The listing builds one solid part. Answer for the finished solid, in the listing's coordinates (mm). A direction names the side the tool comes from. Give positions to 0.01 mm unless a question says otherwise; leave off trailing zeros. Write each loop counter-clockwise with the first axis right and the second up, starting at its lowest first coordinate (ties: lowest second). Pieces come first, ordered by that corner, then holes. Notation, with made-up numbers: (43, -21.75) -> (81, -21.75) arc R26 cw to (81, 14.25) -> close; hole circle Ø7 at (4, -32.75). An arc over 180 degrees is marked (long way). Put each result on its own line as item: value. Start each with the question number.
1) For faces 3 (the flat face through (378.107, 102.08, 85.404)), 4 (the cylindrical face through (466.41, 102.92, 207.94)), 5 (the cylindrical face through (453.3, 102.08, 231.05)), determine the directions among +Z, -Z, +X, -X, +Y, -Y from which every point of the face is accessible in a straight line to the end or side of a thin tool.
2) A cutting plane is placed at D-D (y = 23). Write down the section's boundary in (x, z).
3) A cutting plane is placed at C-C (x = 663.5). Write down the section's boundary in (y, z), then the cut area to 3 significant figures.
4) For a pull along Y with two mould halves and no side action, classify faces 1 (the flat face through (-300, 75, 101)), 2 (the flat face through (423, 132.5, 120)) as released by +Y, released by -Y, zero draft, split by the parting line, or undercut.
5) A cutting plane is placed at A-A (y = 114.5). Give the number of separate pieces and of enclosed holes in the cut face, then the cut area to 3 significant figures.
6) A cutting plane is placed at B-B (z = 232.5). Write down the section's boundary in (x, y).
7) Flat-ended cylindrical pins translate along their axes: pin 1 Ø22 at (x, y) = (556.5, 144.5) entering from -Z; pin 2 Ø4 at (y, z) = (72, 204) entering from -X; pin 3 Ø18 at (x, y) = (586, 106) entering from -Z. Find the tip coordinate at first contact, or state that the pin passes through.
8) Find the intervals of material crossed by line 1 along Y through (x, z) = (500, 195.5); line 2 along X through (y, z) = (118.5, 232.5); line 3 along Z through (x, y) = (652, 66), in increasing order. Write a range as from..to.
from build123d import *

# Parameters (mm, degrees)
BOSS_EXTRUDE1_DEPTH = 152.5
CUT_EXTRUDE1_DEPTH  = 153.5
CUT_EXTRUDE2_REACH  = 154.5
SKETCH7_R           = 35


with BuildPart() as part:
    # Sketch1 → Boss-Extrude1 (new body)
    with BuildSketch(Plane(origin=(0, 0, 0), x_dir=(1, 0, 0), z_dir=(0, 1, 0))):
        with BuildLine():
            Line((-300, -132.5), (-132.5, -132.5))
            ThreePointArc((-132.5, -132.5), (-38.808351493, -93.691648507), (0, 0))
            Line((0, 0), (0, 209.763098819))
            ThreePointArc((0, 209.763098819), (-38.808351493, 303.454747326), (-132.5, 342.263098819))
            Line((-132.5, 342.263098819), (-300, 342.263098819))
            Line((-300, 342.263098819), (-300, 279.881549409))
            Line((-300, 279.881549409), (-125, 104.881549409))
            Line((-125, 104.881549409), (-300, -70.118450591))
            Line((-300, -70.118450591), (-300, -132.5))
        make_face()
    extrude(amount=BOSS_EXTRUDE1_DEPTH)

    # Sketch2 → Cut-Extrude1 (cut, through all)
    with BuildSketch(Plane(origin=(0, 152.5, 0), x_dir=(1, 0, 0), z_dir=(0, 1, 0))):
        with BuildLine():
            Line((-223.447835998, -46.182307711), (-139.361825834, 46.305891731))
            ThreePointArc((-139.361825834, 46.305891731), (-95.697655057, 48.504400086), (-93.258215037, 4.853026901))
            Line((-93.258215037, 4.853026901), (-176.318308109, -88.557599262))
            ThreePointArc((-176.318308109, -88.557599262), (-221.187968417, -91.065122785), (-223.447835998, -46.182307711))
        make_face()
        with BuildLine():
            Line((-93.258215037, 204.910071918), (-176.318308109, 298.320698081))
            ThreePointArc((-176.318308109, 298.320698081), (-221.187968417, 300.828221603), (-223.447835998, 255.94540653))
            Line((-223.447835998, 255.94540653), (-139.361825834, 163.457207088))
            ThreePointArc((-139.361825834, 163.457207088), (-95.697655057, 161.258698732), (-93.258215037, 204.910071918))
        make_face()
    extrude(amount=-CUT_EXTRUDE1_DEPTH, mode=Mode.SUBTRACT)

    # Sweep2: sweep along a path in Sketch4
    with BuildLine(Plane(origin=(0, 0, 0), x_dir=(1, 0, 0), z_dir=(0, 1, 0))) as sweep2_path:
        Line((0, 104.881549409), (125, 104.881549409))
        ThreePointArc((125, 104.881549409), (229.686421658, 77.6733307), (307.876740467, 2.935066808))
        Line((307.876740467, 2.935066808), (424.108620349, -185.083031348))
        ThreePointArc((424.108620349, -185.083031348), (460.476210492, -219.845014554), (509.167569403, -232.5))
        Line((509.167569403, -232.5), (654.167569403, -232.5))
    # Sketch3 → Sweep2 (sweep)
    with BuildSketch(Plane(origin=(0, 0, 0), x_dir=(0, 0, -1), z_dir=(1, 0, 0))):
        Polygon((67.381549409, 152.5), (142.381549409, 152.5), (142.381549409, 132.5), (118.166896534, 132.5), (118.166896534, 72.5), (142.381549409, 72.5), (142.381549409, 52.5), (67.381549409, 52.5), (67.381549409, 72.5), (91.596202285, 72.5), (91.596202285, 132.5), (67.381549409, 132.5), align=None)
    sweep(path=sweep2_path.line)

    # Sketch6 → Revolve2 (revolve)
    with BuildSketch(Plane.XY.offset(232.5)):
        Polygon((654.167569403, 152.5), (574.167569403, 152.5), (574.167569403, 132.5), (614.167569403, 132.5), (614.167569403, 72.5), (574.167569403, 72.5), (574.167569403, 52.5), (654.167569403, 52.5), align=None)
    revolve(axis=Axis((654.167569403, 152.5, 232.5), (0, 1, 0)))

    # Sketch7 → Cut-Extrude2 (cut, up to next)
    with BuildSketch(Plane(origin=(0, 152.5, 0), x_dir=(1, 0, 0), z_dir=(0, 1, 0)), mode=Mode.PRIVATE) as cut_extrude2_sk1:
        with Locations((654.167569403, -232.5)):
            Circle(SKETCH7_R)
    cut_extrude2_tool1 = extrude(cut_extrude2_sk1.sketch, amount=-CUT_EXTRUDE2_REACH, mode=Mode.PRIVATE) & part.part
    add(cut_extrude2_tool1.solids().sort_by_distance((654.167569, 152.5, 232.5))[0], mode=Mode.SUBTRACT)


solid = part.part
Reply:
1. face 3: -Z, +X
1. face 4: -Z
1. face 5: +Z, -X
2. outline: (-300, -342.26) -> (-132.5, -342.26) arc R132.5 ccw to (0, -209.76) -> (0, 0) arc R132.5 ccw to (-132.5, 132.5) -> (-300, 132.5) -> (-300, 70.12) -> (-125, -104.88) -> (-300, -279.88) -> close; hole (-223.45, -255.95) arc R31.69 ccw (long way) to (-176.32, -298.32) -> (-93.26, -204.91) arc R31 ccw to (-139.36, -163.46) -> close; hole (-223.45, 46.18) -> (-139.36, -46.31) arc R31 ccw to (-93.26, -4.85) -> (-176.32, 88.56) arc R31.69 ccw (long way) to start
3. outline: (52.5, 153.05) -> (72.5, 153.05) -> (72.5, 193.6) -> (132.5, 193.6) -> (132.5, 153.05) -> (152.5, 153.05) -> (152.5, 198.77) -> (52.5, 198.77) -> close; (52.5, 266.23) -> (152.5, 266.23) -> (152.5, 311.95) -> (132.5, 311.95) -> (132.5, 271.4) -> (72.5, 271.4) -> (72.5, 311.95) -> (52.5, 311.95) -> close
3. area: 4,280 mm2
4. face 1: zero draft
4. face 2: undercut
5. separate pieces: 1
5. enclosed holes: 3
5. area: 104,000 mm2
6. outline: (414.79, 52.5) -> (619.17, 52.5) -> (619.17, 152.5) -> (414.79, 152.5) -> (414.79, 132.5) -> (455.94, 132.5) -> (455.94, 72.5) -> (414.79, 72.5) -> close; (689.17, 52.5) -> (734.17, 52.5) -> (734.17, 72.5) -> (694.17, 72.5) -> (694.17, 132.5) -> (734.17, 132.5) -> (734.17, 152.5) -> (689.17, 152.5) -> close
7. pin 1: stops at z = 195
7. pin 2: stops at x = 390.48
7. pin 3: stops at z = 219.21
8. line 1: y = 52.5..72.5, 132.5..152.5
8. line 2: x = 455.94..619.17, 689.17..694.17
8. line 3: z = 152.53..197.57, 267.43..312.47
